```python
from build123d import *

# Parameters (mm, degrees)
TAGLIO_ESTRUSIONE1_DEPTH      = 11
TAGLIO_ESTRUSIONE1_DEPTH_BACK = 11
SCHIZZO2_W                    = 63
SCHIZZO2_H                    = 14
RACCORDO1_R                   = 0.5
RACCORDO2_R                   = 11
ESTRUSIONE_ESTRUSIONE1_START  = 30
SCHIZZO3_R                    = 42.5
ESTRUSIONE_ESTRUSIONE1_DEPTH  = 30
SCHIZZO4_R                    = 42.5
ESTRUSIONE_ESTRUSIONE2_DEPTH  = 12
RACCORDO3_R                   = 2
SMUSSO1_SIZE                  = 1


with BuildPart() as part:
    # Schizzo1 → Rivoluzione1 (revolve)
    with BuildSketch(Plane.XY, mode=Mode.PRIVATE) as rivoluzione1_sk:
        Polygon((0, 0), (0, 42.5), (165.5, 42.5), (165.5, 57.5), (188, 57.5), (188, 42.5), (378.5, 42.5), (378.5, 0), align=None)
    revolve(rivoluzione1_sk.sketch.rotate(Axis((-146.856788593, 0, 0), (1, 0, 0)), 90), axis=Axis((-146.856788593, 0, 0), (1, 0, 0)))

    # Schizzo2 → Taglio-Estrusione1 (cut, two sides: drawn at the far end of the back side and taken through both)
    with BuildSketch(Plane.XY.offset(-TAGLIO_ESTRUSIONE1_DEPTH_BACK)):
        with Locations((118, 40.5)):
            Rectangle(SCHIZZO2_W, SCHIZZO2_H)
        with Locations((248, 40.5)):
            Rectangle(SCHIZZO2_W, SCHIZZO2_H)
    extrude(amount=TAGLIO_ESTRUSIONE1_DEPTH + TAGLIO_ESTRUSIONE1_DEPTH_BACK, mode=Mode.SUBTRACT)

    # Raccordo1
    raccordo1_edges = [part.edges().sort_by_distance(p)[0] for p in [
        (149.5, 33.5, 0),
        (118, 33.5, 11),
        (86.5, 33.5, 0),
        (118, 33.5, -11),
        (279.5, 33.5, 0),
        (248, 33.5, 11),
        (216.5, 33.5, 0),
        (248, 33.5, -11),
    ]]
    fillet(raccordo1_edges, radius=RACCORDO1_R)

    # Raccordo2
    # the kernel refuses this fillet: 11 mm, written as the material it adds along each edge
    with BuildSketch(Plane(origin=(268.5, 33.5, 0), x_dir=(0, 0, -1), z_dir=(-1, 0, 0))) as raccordo2_piece_1:
        with BuildLine():
            CenterArc((10.5, -0.5), 0.5, 0, 90)
            Line((11, -0.5), (11, 0))
            Line((11, 0), (10.5, 0))
        make_face()
    revolve(axis=Axis((268.5, 33.5, 0), (0, -1, 0)), revolution_arc=90)
    with BuildSketch(Plane(origin=(268.5, 33.5, 0), x_dir=(1, 0, 0), z_dir=(0, 0, -1))) as raccordo2_piece_2:
        with BuildLine():
            CenterArc((10.5, -0.5), 0.5, 0, 90)
            Line((11, -0.5), (11, 0))
            Line((11, 0), (10.5, 0))
        make_face()
    revolve(axis=Axis((268.5, 33.5, 0), (0, -1, 0)), revolution_arc=90)
    with BuildSketch(Plane(origin=(227.5, 33.5, 0), x_dir=(0, 0, 1), z_dir=(1, 0, 0))) as raccordo2_piece_3:
        with BuildLine():
            CenterArc((10.5, -0.5), 0.5, 0, 90)
            Line((11, -0.5), (11, 0))
            Line((11, 0), (10.5, 0))
        make_face()
    revolve(axis=Axis((227.5, 33.5, 0), (0, -1, 0)), revolution_arc=90)
    with BuildSketch(Plane(origin=(227.5, 33.5, 0), x_dir=(-1, 0, 0), z_dir=(0, 0, 1))) as raccordo2_piece_4:
        with BuildLine():
            CenterArc((10.5, -0.5), 0.5, 0, 90)
            Line((11, -0.5), (11, 0))
            Line((11, 0), (10.5, 0))
        make_face()
    revolve(axis=Axis((227.5, 33.5, 0), (0, -1, 0)), revolution_arc=90)
    with BuildSketch(Plane(origin=(138.5, 33.5, 0), x_dir=(1, 0, 0), z_dir=(0, 0, -1))) as raccordo2_piece_5:
        with BuildLine():
            CenterArc((10.5, -0.5), 0.5, 0, 90)
            Line((11, -0.5), (11, 0))
            Line((11, 0), (10.5, 0))
        make_face()
    revolve(axis=Axis((138.5, 33.5, 0), (0, -1, 0)), revolution_arc=90)
    with BuildSketch(Plane(origin=(138.5, 33.5, 0), x_dir=(0, 0, -1), z_dir=(-1, 0, 0))) as raccordo2_piece_6:
        with BuildLine():
            CenterArc((10.5, -0.5), 0.5, 0, 90)
            Line((11, -0.5), (11, 0))
            Line((11, 0), (10.5, 0))
        make_face()
    revolve(axis=Axis((138.5, 33.5, 0), (0, -1, 0)), revolution_arc=90)
    with BuildSketch(Plane(origin=(97.5, 33.5, 0), x_dir=(0, 0, 1), z_dir=(1, 0, 0))) as raccordo2_piece_7:
        with BuildLine():
            CenterArc((10.5, -0.5), 0.5, 0, 90)
            Line((11, -0.5), (11, 0))
            Line((11, 0), (10.5, 0))
        make_face()
    revolve(axis=Axis((97.5, 33.5, 0), (0, -1, 0)), revolution_arc=90)
    with BuildSketch(Plane(origin=(97.5, 33.5, 0), x_dir=(-1, 0, 0), z_dir=(0, 0, 1))) as raccordo2_piece_8:
        with BuildLine():
            CenterArc((10.5, -0.5), 0.5, 0, 90)
            Line((11, -0.5), (11, 0))
            Line((11, 0), (10.5, 0))
        make_face()
    revolve(axis=Axis((97.5, 33.5, 0), (0, -1, 0)), revolution_arc=90)
    with BuildSketch(Plane(origin=(86.5, 33.5, -11), x_dir=(0, 0, 1), z_dir=(0, 1, 0))) as raccordo2_piece_9_section:
        with BuildLine():
            CenterArc((RACCORDO2_R, RACCORDO2_R), RACCORDO2_R, 180, 90)
            Line((0, RACCORDO2_R), (0, 0))
            Line((0, 0), (RACCORDO2_R, 0))
        make_face()
    raccordo2_piece_9 = extrude(amount=35.05179655, mode=Mode.PRIVATE)
    raccordo2_piece_9 = raccordo2_piece_9 & Plane(origin=(88.913570228, 0, 0), x_dir=(0, 0, 1), z_dir=(1, 0, 0)) * Cylinder(42.5, 115, mode=Mode.PRIVATE)
    add(raccordo2_piece_9)
    with BuildSketch(Plane(origin=(86.5, 33.5, 11), x_dir=(0, 0, -1), z_dir=(0, 1, 0))) as raccordo2_piece_10_section:
        with BuildLine():
            CenterArc((RACCORDO2_R, -RACCORDO2_R), RACCORDO2_R, 90, 90)
            Line((0, -RACCORDO2_R), (0, 0))
            Line((0, 0), (RACCORDO2_R, 0))
        make_face()
    raccordo2_piece_10 = extrude(amount=35.05179655, mode=Mode.PRIVATE)
    raccordo2_piece_10 = raccordo2_piece_10 & Plane(origin=(88.913567526, 0, 0), x_dir=(0, 0, 1), z_dir=(1, 0, 0)) * Cylinder(42.5, 115, mode=Mode.PRIVATE)
    add(raccordo2_piece_10)
    with BuildSketch(Plane(origin=(149.5, 68.55179655, -11), x_dir=(-1, 0, 0), z_dir=(0, -1, 0))) as raccordo2_piece_11_section:
        with BuildLine():
            CenterArc((RACCORDO2_R, -RACCORDO2_R), RACCORDO2_R, 90, 90)
            Line((0, -RACCORDO2_R), (0, 0))
            Line((0, 0), (RACCORDO2_R, 0))
        make_face()
    raccordo2_piece_11 = extrude(amount=35.05179655, mode=Mode.PRIVATE)
    raccordo2_piece_11 = raccordo2_piece_11 & Plane(origin=(147.086427886, 0, 0), x_dir=(0, 0, 1), z_dir=(1, 0, 0)) * Cylinder(42.5, 115, mode=Mode.PRIVATE)
    add(raccordo2_piece_11)
    with BuildSketch(Plane(origin=(149.5, 68.55179655, 11), x_dir=(-1, 0, 0), z_dir=(0, -1, 0))) as raccordo2_piece_12_section:
        with BuildLine():
            CenterArc((RACCORDO2_R, RACCORDO2_R), RACCORDO2_R, 180, 90)
            Line((0, RACCORDO2_R), (0, 0))
            Line((0, 0), (RACCORDO2_R, 0))
        make_face()
    raccordo2_piece_12 = extrude(amount=35.05179655, mode=Mode.PRIVATE)
    raccordo2_piece_12 = raccordo2_piece_12 & Plane(origin=(147.086433525, 0, 0), x_dir=(0, 0, 1), z_dir=(1, 0, 0)) * Cylinder(42.5, 115, mode=Mode.PRIVATE)
    add(raccordo2_piece_12)
    with BuildSketch(Plane(origin=(216.5, 33.5, -11), x_dir=(0, 0, 1), z_dir=(0, 1, 0))) as raccordo2_piece_13_section:
        with BuildLine():
            CenterArc((RACCORDO2_R, RACCORDO2_R), RACCORDO2_R, 180, 90)
            Line((0, RACCORDO2_R), (0, 0))
            Line((0, 0), (RACCORDO2_R, 0))
        make_face()
    raccordo2_piece_13 = extrude(amount=35.05179655, mode=Mode.PRIVATE)
    raccordo2_piece_13 = raccordo2_piece_13 & Plane(origin=(218.913570228, 0, 0), x_dir=(0, 0, 1), z_dir=(1, 0, 0)) * Cylinder(42.5, 115, mode=Mode.PRIVATE)
    add(raccordo2_piece_13)
    with BuildSketch(Plane(origin=(216.5, 33.5, 11), x_dir=(0, 0, -1), z_dir=(0, 1, 0))) as raccordo2_piece_14_section:
        with BuildLine():
            CenterArc((RACCORDO2_R, -RACCORDO2_R), RACCORDO2_R, 90, 90)
            Line((0, -RACCORDO2_R), (0, 0))
            Line((0, 0), (RACCORDO2_R, 0))
        make_face()
    raccordo2_piece_14 = extrude(amount=35.05179655, mode=Mode.PRIVATE)
    raccordo2_piece_14 = raccordo2_piece_14 & Plane(origin=(218.913567526, 0, 0), x_dir=(0, 0, 1), z_dir=(1, 0, 0)) * Cylinder(42.5, 115, mode=Mode.PRIVATE)
    add(raccordo2_piece_14)
    with BuildSketch(Plane(origin=(279.5, 68.55179655, 11), x_dir=(-1, 0, 0), z_dir=(0, -1, 0))) as raccordo2_piece_15_section:
        with BuildLine():
            CenterArc((RACCORDO2_R, RACCORDO2_R), RACCORDO2_R, 180, 90)
            Line((0, RACCORDO2_R), (0, 0))
            Line((0, 0), (RACCORDO2_R, 0))
        make_face()
    raccordo2_piece_15 = extrude(amount=35.05179655, mode=Mode.PRIVATE)
    raccordo2_piece_15 = raccordo2_piece_15 & Plane(origin=(277.086433525, 0, 0), x_dir=(0, 0, 1), z_dir=(1, 0, 0)) * Cylinder(42.5, 115, mode=Mode.PRIVATE)
    add(raccordo2_piece_15)
    with BuildSketch(Plane(origin=(279.5, 68.55179655, -11), x_dir=(0, 0, 1), z_dir=(0, -1, 0))) as raccordo2_piece_16_section:
        with BuildLine():
            CenterArc((RACCORDO2_R, RACCORDO2_R), RACCORDO2_R, 180, 90)
            Line((0, RACCORDO2_R), (0, 0))
            Line((0, 0), (RACCORDO2_R, 0))
        make_face()
    raccordo2_piece_16 = extrude(amount=35.05179655, mode=Mode.PRIVATE)
    raccordo2_piece_16 = raccordo2_piece_16 & Plane(origin=(277.086429772, 0, 0), x_dir=(0, 0, 1), z_dir=(1, 0, 0)) * Cylinder(42.5, 115, mode=Mode.PRIVATE)
    add(raccordo2_piece_16)

    # Schizzo3 → Estrusione-Estrusione1 (add)
    with BuildSketch(Plane(origin=(378.5, 0, 0), x_dir=(0, 0, -1), z_dir=(1, 0, 0)).offset(ESTRUSIONE_ESTRUSIONE1_START)):
        with Locations(Location((0, 0, 0), (0, 0, 180))):
            Circle(SCHIZZO3_R)
    extrude(amount=-ESTRUSIONE_ESTRUSIONE1_DEPTH)

    # Schizzo4 → Estrusione-Estrusione2 (add)
    with BuildSketch(Plane.ZY):
        Circle(SCHIZZO4_R)
    extrude(amount=ESTRUSIONE_ESTRUSIONE2_DEPTH)

    # Raccordo3
    raccordo3_edges = [part.edges().sort_by_distance(p)[0] for p in [
        (188, 0, -42.5),
        (165.5, 0, -42.5),
    ]]
    fillet(raccordo3_edges, radius=RACCORDO3_R)

    # Smusso1
    smusso1_edges = [part.edges().sort_by_distance(p)[0] for p in [
        (408.5, 0, -42.5),
        (-12, 0, -42.5),
    ]]
    chamfer(smusso1_edges, length=SMUSSO1_SIZE)


solid = part.part
```
Work out the finished part from the listing and answer in its coordinate system (mm). A direction names the side the tool comes from. Give positions to 0.01 mm unless a question says otherwise; leave off trailing zeros. Order: outer loops, then holes, each group sorted by start corner. A loop starts at its lowest first (then second) coordinate and runs counter-clockwise, first axis right, second up. Notation, with made-up numbers: M 14,-14 L 27,-14 A34 ccw 27,18 Z; hole C -30.75,11.25 d3. An arc over 180 degrees is marked long. Return JSON: item names as keys, results as strings.
1) A tool of negligible diameter and unlimited length cuts with its end or side. For faces 1 (the flat face through (165.5, 34, -30)), 2 (the cylindrical face through (176.908, 56.133, -12.465)), 3 (the flat face through (188, 34, 30)), 4 (the flat face through (118, 38, 11)), 5 (the flat face through (-12, 1, -1)), from which of +Z, -Z, +X, -X, +Y, -Y can it reach the whole face along a straight path? Write none if from no direction.
Resolved:
{"face 1": "-X", "face 2": "+X, -X", "face 3": "+X", "face 4": "+Y", "face 5": "+Z, -Z, -X, +Y, -Y"}
2) Each of these flat-tipped pins is pushed along its axis until it touches: pin 1 (8 mm diameter, centred on x = 264.5, y = -23.5, fed in from +Z); pin 2 (10 mm diameter, centred on x = 43, y = -1, fed in from +Z); pin 3 (10.5 mm diameter, centred on x = 126, z = -1, fed in from +Y). Where does it stop, or does it pass through?
Resolved:
{"pin 1": "z = 37.76", "pin 2": "z = 42.5", "pin 3": "y = 33.5"}
3) Straight lines are drawn through the part: line 1 along X through (y, z) = (38, -5.5); line 2 along X through (y, z) = (-46, -17.5); line 3 along X through (y, z) = (29, -33). For each, find the intervals that lie inside material, in ascending order. Write a range as [from, to].
Resolved:
{"line 1": "[-12, 87.97], [148.03, 217.97], [278.03, 408.5]", "line 2": "[165.5, 188]", "line 3": "[165.42, 188.08]"}
4) Section A-A, the plane y = 0 is taken. Write down the section's boundary in (x, z).
Resolved:
{"outline": "M -12,-41.5 L -11,-42.5 L 163.5,-42.5 A2 cw 165.5,-44.5 L 165.5,-57.5 L 188,-57.5 L 188,-44.5 A2 cw 190,-42.5 L 407.5,-42.5 L 408.5,-41.5 L 408.5,41.5 L 407.5,42.5 L 190,42.5 A2 cw 188,44.5 L 188,57.5 L 165.5,57.5 L 165.5,44.5 A2 cw 163.5,42.5 L -11,42.5 L -12,41.5 Z"}
5) Section D-D, the plane x = 317 is taken. Write down the section's boundary in (y, z), plus the area to 3 significant figures.
Resolved:
{"outline": "C 0,0 d85", "area": "5,670 mm^2"}
6) Section B-B, the plane x = 247 is taken. Write down the section's boundary in (y, z), plus the area to 3 significant figures.
Resolved:
{"outline": "M 33.5,-10.5 L 33.5,10.5 A0.5 cw 34,11 L 41.05,11 A42.5 ccw long 41.05,-11 L 34,-11 A0.5 cw Z", "area": "5,490 mm^2"}
